```python
from build123d import *

# Parameters (mm, degrees)
BOSS_EXTRUDE2_DEPTH   = 23
SKETCH1_W             = 20.789980378
SKETCH1_H             = 6
BOSS_EXTRUDE2_2_DEPTH = 23
BOSS_EXTRUDE2_3_DEPTH = 23
BOSS_EXTRUDE2_4_DEPTH = 23
SKETCH1_3_W           = 20.789980378
SKETCH1_3_H           = 36.5
BOSS_EXTRUDE3_DEPTH   = 11
BOSS_EXTRUDE5_DEPTH   = 45
SKETCH2_W             = 9
SKETCH2_H             = 8
CUT_EXTRUDE1_DEPTH    = 106.353028551
SKETCH3_W             = 24.5
SKETCH3_H             = 11
BOSS_EXTRUDE6_DEPTH   = 42
BOSS_EXTRUDE7_DEPTH   = 11
CHAMFER2_SIZE         = 10


with BuildPart() as part:
    # Sketch1 → Boss-Extrude2 (new body)
    with BuildSketch(Plane(origin=(0, 0, 0), x_dir=(1, 0, 0), z_dir=(0, 1, 0))):
        Polygon((0.945063883, 6), (0.945063883, 0), (1.890127766, 0), (21.735044261, 0), (21.735044261, 6), align=None)
    extrude(amount=BOSS_EXTRUDE2_DEPTH)



with BuildPart() as body_2:
    # Sketch1 → Boss-Extrude2 2 (new body)
    with BuildSketch(Plane(origin=(0, 0, 0), x_dir=(1, 0, 0), z_dir=(0, 1, 0))):
        with Locations((11.340054072, -15.5)):
            Rectangle(SKETCH1_W, SKETCH1_H)
    extrude(amount=BOSS_EXTRUDE2_2_DEPTH)


with BuildPart() as body_3:
    # Sketch1 → Boss-Extrude2 3 (new body)
    with BuildSketch(Plane(origin=(0, 0, 0), x_dir=(1, 0, 0), z_dir=(0, 1, 0))):
        with Locations((54.13003445, -15.5)):
            Rectangle(SKETCH1_W, SKETCH1_H)
    extrude(amount=BOSS_EXTRUDE2_3_DEPTH)


with BuildPart() as body_4:
    # Sketch1 → Boss-Extrude2 4 (new body)
    with BuildSketch(Plane(origin=(0, 0, 0), x_dir=(1, 0, 0), z_dir=(0, 1, 0))):
        with Locations((54.13003445, 3)):
            Rectangle(SKETCH1_W, SKETCH1_H)
    extrude(amount=BOSS_EXTRUDE2_4_DEPTH)


with BuildPart() as part_1:
    add(part.part)

    add(body_2.part)  # Boss-Extrude3 merges body 2
    # Sketch1<3> → Boss-Extrude3 (add)
    with BuildSketch(Plane(origin=(0, 0, 0), x_dir=(1, 0, 0), z_dir=(0, 1, 0))):
        with Locations((11.340054072, -12.25)):
            Rectangle(SKETCH1_3_W, SKETCH1_3_H)
        with Locations((54.13003445, -12.25)):
            Rectangle(SKETCH1_3_W, SKETCH1_3_H)
    extrude(amount=-BOSS_EXTRUDE3_DEPTH)

    # Sketch1<6> → Boss-Extrude5 (add)
    with BuildSketch(Plane(origin=(0, 0, 0), x_dir=(1, 0, 0), z_dir=(0, 1, 0))):
        Polygon((43.735044261, -18.5), (32.735044261, -18.5), (32.735044261, -60.5), (43.735044261, -60.5), (43.735044261, -30.5), align=None)
        Polygon((32.735044261, -18.5), (21.735044261, -18.5), (21.735044261, -30.5), (21.735044261, -60.5), (32.735044261, -60.5), align=None)
    extrude(amount=-BOSS_EXTRUDE5_DEPTH)

    # Sketch2 → Cut-Extrude1 (cut, through all)
    with BuildSketch(Plane(origin=(74.525024639, 0, 0), x_dir=(0, 0, -1), z_dir=(1, 0, 0))):
        Polygon((-30.5, -11), (-30.5, -3), (-41.183889214, -3), (-57.5, -3), (-57.5, -14.989659462), (-57.5, -41), (-21.5, -41), (-21.5, -11), align=None)
        with Locations((-26, -7)):
            Rectangle(SKETCH2_W, SKETCH2_H)
    extrude(amount=-CUT_EXTRUDE1_DEPTH, mode=Mode.SUBTRACT)


    add(body_3.part)  # Boss-Extrude6 merges body 3

    add(body_4.part)  # Boss-Extrude6 merges body 4
    # Sketch3 → Boss-Extrude6 (add)
    with BuildSketch(Plane.ZY.offset(-43.735044261)):
        with Locations((6.25, -5.5)):
            Rectangle(SKETCH3_W, SKETCH3_H)
    extrude(amount=BOSS_EXTRUDE6_DEPTH)

    # Sketch4 → Boss-Extrude7 (add)
    with BuildSketch(Plane(origin=(0, 0, 0), x_dir=(1, 0, 0), z_dir=(0, 1, 0))):
        Polygon((64.525024639, -18.5), (43.735044261, -18.5), (43.735044261, -12.5), (64.525024639, -12.5), (64.525024639, 0), (43.735044261, 0), (43.735044261, 6), (21.735044261, 6), (21.735044261, 0), (0.945063883, 0), (0.945063883, -12.5), (21.735044261, -12.5), (21.735044261, -18.5), (0.945063883, -18.5), (0.945063883, -30.5), (21.735044261, -30.5), (21.735044261, -60.5), (43.735044261, -60.5), (43.735044261, -30.5), (64.525024639, -30.5), align=None)
    extrude(amount=BOSS_EXTRUDE7_DEPTH)

    # Chamfer2
    chamfer2_edges = [part_1.edges().sort_by_distance(p)[0] for p in [
        (11.340054072, 11, 30.5),
        (32.735044261, 11, 60.5),
        (54.13003445, 11, 30.5),
    ]]
    chamfer(chamfer2_edges, length=CHAMFER2_SIZE)


solid = part_1.part
```
CAD build for the part. Positions are in the model's coordinates, mm. A direction names the side the tool comes from. Give positions to 0.01 mm unless a question says otherwise; leave off trailing zeros. Loops run counter-clockwise (first coordinate to the right, second up) from the corner with the lowest first, then second, coordinate; pieces in that order, holes last. Notation, with made-up numbers: (70.25, 49.25) -> (105.25, 49.25) arc R12 ccw to (105.25, 54.25) -> close; hole circle Ø6 at (12.25, -2). An arc over 180 degrees is marked (long way). Use a Markdown table: item, result.
1. Wall check: L1, parallel to Z at x = 33.5, y = -24; L2, parallel to Z at x = 51, y = 13.5; L3, parallel to Y at x = 45.5, z = 19. Give the ranges that are in metal, low to high. Write a range as [from, to].
Check result:
| item | result |
|---|---|
| L1 | z = [18.5, 21.5], [57.5, 60.5] |
| L2 | z = [-6, 0], [12.5, 18.5] |
| L3 | y = [-11, 11] |
2. Slice it at C-C (x = 55). List the corners of the cut face in (y, z).
Check result:
| item | result |
|---|---|
| outline | (-11, -6) -> (23, -6) -> (23, 0) -> (11, 0) -> (11, 12.5) -> (23, 12.5) -> (23, 18.5) -> (11, 18.5) -> (11, 20.5) -> (1, 30.5) -> (-3, 30.5) -> (-3, 21.5) -> (-11, 21.5) -> close |
3. Which spindle directions (+Z, -Z, +X, -X, +Y, -Y) get a long thin tool onto all of the face, cutting with end or side? Do faces 4 (the flat face through (33, -28, 18.5)), 5 (the flat face through (33, -22, 57.5)), 6 (the flat face through (43.735, 17, 16)), 7 (the flat face through (11, 17, 12.5)), 8 (the flat face through (11, -1, 30.5)). Say none if no direction does.
Check result:
| item | result |
|---|---|
| face 4 | -Z, +X, -X, -Y |
| face 5 | +X, -X |
| face 6 | +Z, -Z, +Y |
| face 7 | +X, -X, +Y |
| face 8 | +Z, -X, +Y, -Y |
4. Slice it at B-B (z = 43). List the corners of the cut face in (x, y).
Check result:
| item | result |
|---|---|
| outline | (21.74, -45) -> (43.74, -45) -> (43.74, -41) -> (21.74, -41) -> close; (21.74, -3) -> (43.74, -3) -> (43.74, 11) -> (21.74, 11) -> close |
5. Slice it at D-D (y = 5.5). List the corners of the cut face in (x, z).
Check result:
| item | result |
|---|---|
| outline | (0.95, -6) -> (64.53, -6) -> (64.53, 26) -> (43.74, 26) -> (43.74, 56) -> (21.74, 56) -> (21.74, 26) -> (0.95, 26) -> close |
6. Slice it at A-A (y = -9.5). List the corners of the cut face in (x, z), plus the area to 3 significant figures.
Check result:
| item | result |
|---|---|
| outline | (0.95, -6) -> (64.53, -6) -> (64.53, 21.5) -> (0.95, 21.5) -> close; (21.74, 57.5) -> (43.74, 57.5) -> (43.74, 60.5) -> (21.74, 60.5) -> close |
| area | 1,810 mm^2 |
7. Flat gauge pins, fed straight in: pin 1 (2 mm diameter, centred on x = 58, z = 8.5, fed in from +Y); pin 2 (21 mm diameter, centred on y = -20, z = 31, fed in from -X); pin 3 (5 mm diameter, centred on y = -22.5, z = 20, fed in from +X). Where does each tip first touch, or does it go through?
Check result:
| item | result |
|---|---|
| pin 1 | stops at y = 11 |
| pin 2 | stops at x = 21.74 |
| pin 3 | stops at x = 43.74 |
8. Mould opens along Y. For faces 1 (the flat face through (33, -18, 21.5)), 2 (the flat face through (21.735, 17, -3)), 3 (the flat face through (54, 6.1, 25.4)) say: pulls with the +Y half, pulls with the -Y half, needs draft (parallel to the pull), parting line crosses it, or undercut.
Check result:
| item | result |
|---|---|
| face 1 | undercut |
| face 2 | needs draft |
| face 3 | pulls with the +Y half |
